```python
from build123d import *

# Parameters (mm, degrees)
F0_R           = 25.5
F1_DEPTH       = 10
F0_R_2         = 7.5
F2_DEPTH       = 5
F4_D           = 3
F4_DEPTH       = 11
F4_CSINK_D     = 5
F4_CSINK_ANGLE = 90


with BuildPart() as f1:
    # F0 (on Top) → F1 (new body)
    with BuildSketch(Plane.XY):
        with BuildLine():
            Line((21.5, 26.5), (-21.5, 26.5))
            ThreePointArc((-21.5, 26.5), (-25.035534, 25.035534), (-26.5, 21.5))
            Line((-26.5, 21.5), (-26.5, -21.5))
            ThreePointArc((-26.5, -21.5), (-25.035534, -25.035534), (-21.5, -26.5))
            Line((-21.5, -26.5), (21.5, -26.5))
            ThreePointArc((21.5, -26.5), (25.035534, -25.035534), (26.5, -21.5))
            Line((26.5, -21.5), (26.5, 21.5))
            ThreePointArc((26.5, 21.5), (25.035534, 25.035534), (21.5, 26.5))
        make_face()
        Circle(F0_R, mode=Mode.SUBTRACT)
    extrude(amount=F1_DEPTH)

    # F0 (on Top) → F2 (join)
    with BuildSketch(Plane.XY):
        Circle(F0_R)
        Circle(F0_R_2, mode=Mode.SUBTRACT)
    extrude(amount=F2_DEPTH)

    # F4
    with Locations(Plane(origin=(0, 0, 0), x_dir=(1, 0, 0), z_dir=(0, 0, -1))):
        with Locations((-21.5, 21.5), (-21.5, -21.5), (21.5, -21.5), (21.5, 21.5)):
            CounterSinkHole(F4_D / 2, F4_CSINK_D / 2, depth=F4_DEPTH, counter_sink_angle=F4_CSINK_ANGLE)


solid = f1.part
```
Can you work these out from the model? Positions are in its coordinate system, mm. A direction names the side the tool comes from. Coordinates: 2 decimals unless noted, no trailing zeros. Order: outer loops, then holes, each group sorted by start corner. A loop starts at its lowest first (then second) coordinate and runs counter-clockwise, first axis right, second up. Notation, with made-up numbers: (50, 16.5) - (79, 16.5) arc R18 ccw to (79, 38.5) - close; hole circle Ø1 at (59.25, 66). An arc over 180 degrees is marked (long way). Answer in a Markdown table with one row per item.
1. If we mould it in two halves opening along Y, with no side actions, what happens to faces 1 (the flat face through (-26, 0, 10)), 2 (the cylindrical face through (-25, 25.07, 4.93)), 3 (the flat face through (5, 6, 5))? For each: pulls with the +Y half, pulls with the -Y half, needs draft (parallel to the pull), parting line crosses it, or undercut.
Reply:
| item | result |
|---|---|
| face 1 | needs draft |
| face 2 | pulls with the +Y half |
| face 3 | undercut |
2. Suppose I cut it at D-D (y = 12.5). Please give me the cut outline in (x, z), and give its area (3 significant figures).
Reply:
| item | result |
|---|---|
| outline | (-26.5, 0) - (26.5, 0) - (26.5, 10) - (22.23, 10) - (22.23, 5) - (-22.23, 5) - (-22.23, 10) - (-26.5, 10) - close |
| area | 308 mm^2 |
3. For pin 1 (4 mm diameter, centred on x = -21.5, y = -21.5, fed in from -Z); pin 2 (24 mm diameter, centred on x = 0, y = 0, fed in from +Z), each with a flat end and sliding along its axis, tell me the tip position at first contact or that it passes through.
Reply:
| item | result |
|---|---|
| pin 1 | stops at z = 0.5 |
| pin 2 | stops at z = 5 |
4. For faces 4 (the cylindrical face through (-5.5, -24.9, 7.5)), 5 (the cylindrical face through (-20.39, 20.49, 5.56)), which set-ups out of +Z, -Z, +X, -X, +Y, -Y let a thin tool reach every point of the face, with its end or its side?
Reply:
| item | result |
|---|---|
| face 4 | +Z |
| face 5 | +Z, -Z |
5. If I drill on line 1 along X through (y, z) = (-21.5, 3.5); line 2 along Y through (x, z) = (-21.5, 7.25), over which ranges is the centre line in solid material (lowest first)?
Reply:
| item | result |
|---|---|
| line 1 | x = -26.5 to -23, -20 to 20, 23 to 26.5 |
| line 2 | y = -26.5 to -23, -20 to -13.71, 13.71 to 20, 23 to 26.5 |
6. Suppose I cut it at C-C (z = 6). Please give me the cut outline in (x, y).
Reply:
| item | result |
|---|---|
| outline | (-26.5, -21.5) arc R5 ccw to (-21.5, -26.5) - (21.5, -26.5) arc R5 ccw to (26.5, -21.5) - (26.5, 21.5) arc R5 ccw to (21.5, 26.5) - (-21.5, 26.5) arc R5 ccw to (-26.5, 21.5) - close; hole circle Ø51 at (0, 0); hole circle Ø3 at (-21.5, -21.5); hole circle Ø3 at (-21.5, 21.5); hole circle Ø3 at (21.5, -21.5); hole circle Ø3 at (21.5, 21.5) |
7. Suppose I cut it at A-A (x = 0). Please give me the cut outline in (y, z).
Reply:
| item | result |
|---|---|
| outline | (-26.5, 0) - (-7.5, 0) - (-7.5, 5) - (-25.5, 5) - (-25.5, 10) - (-26.5, 10) - close; (7.5, 0) - (26.5, 0) - (26.5, 10) - (25.5, 10) - (25.5, 5) - (7.5, 5) - close |
